The listing builds one solid part. Answer for the finished solid, in the listing's coordinates (mm). A direction names the side the tool comes from. Give positions to 0.01 mm unless a question says otherwise; leave off trailing zeros. Order: outer loops, then holes, each group sorted by start corner. A loop starts at its lowest first (then second) coordinate and runs counter-clockwise, first axis right, second up. Notation, with made-up numbers: (-16, 61) - (40, 61) arc R20 ccw to (40, 98) - close; hole circle Ø7 at (57.25, 89.5). An arc over 180 degrees is marked (long way). Write each question's results on one line, items separated by ' | '. Start each with the question number.
1. Find the intervals of material crossed by L1, parallel to X at y = 0.7, z = 0; L2, parallel to X at y = 2, z = 0; L3, parallel to Z at x = -8, y = 7.75, in increasing order.
2. Section B-B (y = 6.5) is taken. Give the vertices of the cut face in (x, z).
3. Section D-D (z = 5) is taken. Give the vertices of the cut face in (x, y) (3 decimals), and give its area (3 significant figures).
4. Section A-A (z = 0) is taken. State how many separate pieces and enclosed holes the cut face has, and give its area (3 significant figures).
5. Flat-ended cylindrical pins translate along their axes: pin 1 (1.3 mm diameter, centred on y = 7.5, z = -9.5, fed in from +X); pin 2 (4 mm diameter, centred on y = 5.5, z = 2, fed in from -X); pin 3 (1.3 mm diameter, centred on x = -3, z = -9.5, fed in from +Y) (3 decimals). Find the tip coordinate at first contact, or state that the pin passes through.
6. Section C-C (x = -4) is taken. Give the vertices of the cut face in (y, z) (1 decimal), and give its area (3 significant figures).
7. Which of the six approach directions +Z, -Z, +X, -X, +Y, -Y give full straight-line access (tool end or side, diameter ignored) to faces 1 (the face through (15.589, 8, 0)), 2 (the face through (0, 5, 10.033)), 3 (the face through (8.895, 7.254, -4.934)), 4 (the face through (11, 1.026, 0)), 5 (the face through (6.35, 8, 9))?
8. Determine the mould class of faces 6 (the face through (19, 0, 0)), 7 (the face through (-27.97, 1.288, -9.753)), 8 (the face through (16.353, 3.264, -0.14)), 9 (the face through (25.272, 1.288, 1.172)) for opening direction X: released by +X, released by -X, zero draft, split by the parting line, or undercut.
from build123d import *

# Parameters (mm, degrees)
SKETCH1_W               = 32.0675
SKETCH1_H               = 20.955
BOSS_EXTRUDE2_DEPTH     = 2.54
SKETCH3_W               = 31.1785
SKETCH3_H               = 20.066
SKETCH3_W_2             = 28.0035
SKETCH3_H_2             = 16.891
EXTRUDE_THIN1_DEPTH     = 8.255
CUT_EXTRUDE1_DEPTH      = 29.508335431
CUT_EXTRUDE1_DEPTH_BACK = 29.508335431
SKETCH4_W               = 12.7
SKETCH4_H               = 5.08
SKETCH5_R               = 1.5
BOSS_EXTRUDE3_DEPTH     = 8.255
FILLET1_R               = 1.27
CUT_EXTRUDE2_DEPTH      = 29.508335431
CUT_EXTRUDE2_DEPTH_BACK = 29.508335431
SKETCH6_W               = 3.048
SKETCH6_H               = 1.02616
SKETCH7_W               = 20.955
SKETCH7_H               = 2.54
BOSS_EXTRUDE4_DEPTH     = 12.7
FILLET2_R               = 2.54
FILLET3_R               = 2.54
SKETCH8_R               = 2.54
CUT_EXTRUDE3_DEPTH      = 32.67887972
FILLET4_R               = 2.54


with BuildPart() as part:
    # Sketch1 → Boss-Extrude2 (new body)
    with BuildSketch(Plane(origin=(0, 0, 0), x_dir=(1, 0, 0), z_dir=(0, 1, 0))):
        Rectangle(SKETCH1_W, SKETCH1_H)
    extrude(amount=BOSS_EXTRUDE2_DEPTH)

    # Sketch3 → Extrude-Thin1 (add)
    with BuildSketch(Plane(origin=(0, 2.54, 0), x_dir=(1, 0, 0), z_dir=(0, 1, 0))):
        Rectangle(SKETCH3_W, SKETCH3_H)
        Rectangle(SKETCH3_W_2, SKETCH3_H_2, mode=Mode.SUBTRACT)
    extrude(amount=EXTRUDE_THIN1_DEPTH)

    # Sketch4 → Cut-Extrude1 (cut, two sides: drawn at the far end of the back side and taken through both)
    with BuildSketch(Plane(origin=(0, 0, -10.4775), x_dir=(-1, 0, 0), z_dir=(0, 0, -1)).offset(-CUT_EXTRUDE1_DEPTH_BACK)):
        with Locations((0, 8.255)):
            Rectangle(SKETCH4_W, SKETCH4_H)
    extrude(amount=CUT_EXTRUDE1_DEPTH + CUT_EXTRUDE1_DEPTH_BACK, mode=Mode.SUBTRACT)

    # Sketch5 → Boss-Extrude3 (add)
    with BuildSketch(Plane(origin=(0, 2.54, 0), x_dir=(1, 0, 0), z_dir=(0, 1, 0))):
        with Locations(Location((-10.16, 4.1275, 0), (0, 0, 270))):
            Circle(SKETCH5_R)
        with Locations(Location((10.16, 4.1275, 0), (0, 0, 90))):
            Circle(SKETCH5_R)
    extrude(amount=BOSS_EXTRUDE3_DEPTH)

    # Fillet1
    fillet1_edges = [part.edges().sort_by_distance(p)[0] for p in [
        (-10.16, 2.54, -5.6275),
        (10.16, 2.54, -2.6275),
    ]]
    fillet(fillet1_edges, radius=FILLET1_R)

    # Sketch6 → Cut-Extrude2 (cut, two sides: drawn at the far end of the back side and taken through both)
    with BuildSketch(Plane.XY.offset(10.4775).offset(-CUT_EXTRUDE2_DEPTH_BACK)):
        with Locations((-10.969625, 0.51308)):
            Rectangle(SKETCH6_W, SKETCH6_H)
        with Locations((10.969625, 0.51308)):
            Rectangle(SKETCH6_W, SKETCH6_H)
    extrude(amount=CUT_EXTRUDE2_DEPTH + CUT_EXTRUDE2_DEPTH_BACK, mode=Mode.SUBTRACT)

    # Sketch7 → Boss-Extrude4 (add)
    with BuildSketch(Plane.ZY.offset(16.03375)):
        with Locations((0, 1.27)):
            Rectangle(SKETCH7_W, SKETCH7_H)
    boss_extrude4 = extrude(amount=BOSS_EXTRUDE4_DEPTH)

    # Fillet2
    fillet2_edges = [part.edges().sort_by_distance(p)[0] for p in [
        (-28.73375, 1.27, -10.4775),
        (-28.73375, 1.27, 10.4775),
    ]]
    fillet(fillet2_edges, radius=FILLET2_R)

    # Fillet3
    fillet3_edges = [part.edges().sort_by_distance(p)[0] for p in [
        (-15.58925, 2.54, 0),
    ]]
    fillet(fillet3_edges, radius=FILLET3_R)

    # Sketch8 → Cut-Extrude3 (cut, symmetric)
    with BuildSketch(Plane(origin=(0, 2.54, 0), x_dir=(1, 0, 0), z_dir=(0, 1, 0))):
        with Locations(Location((-23.01875, 0, 0), (0, 0, 270))):
            Circle(SKETCH8_R)
    cut_extrude3 = extrude(amount=CUT_EXTRUDE3_DEPTH, both=True, mode=Mode.SUBTRACT)

    # Mirror2: Boss-Extrude4 across plane
    add(boss_extrude4.mirror(Plane(origin=(0, 0, 0), x_dir=(0, 0, 1), z_dir=(1, 0, 0))))

    # Mirror6: Cut-Extrude3 across plane
    add(cut_extrude3.mirror(Plane(origin=(0, 0, 0), x_dir=(0, 0, 1), z_dir=(1, 0, 0))), mode=Mode.SUBTRACT)

    # Fillet4
    fillet4_edges = [part.edges().sort_by_distance(p)[0] for p in [
        (28.73375, 1.27, -10.4775),
        (28.73375, 1.27, 10.4775),
        (15.58925, 2.54, 0),
    ]]
    fillet(fillet4_edges, radius=FILLET4_R)


solid = part.part
Reported:
1) L1: -28.73 to -25.56, -20.48 to -12.49, -9.45 to 9.45, 12.49 to 20.48, 25.56 to 28.73 | L2: -28.73 to -25.56, -20.48 to 20.48, 25.56 to 28.73 | L3: -10.03 to -8.45, 8.45 to 10.03
2) outline: (-15.59, -10.03) - (-6.35, -10.03) - (-6.35, -8.45) - (-14, -8.45) - (-14, 8.45) - (-6.35, 8.45) - (-6.35, 10.03) - (-15.59, 10.03) - close; circle Ø3 at (-10.16, -4.13); (6.35, -10.03) - (15.59, -10.03) - (15.59, 10.03) - (6.35, 10.03) - (6.35, 8.45) - (14, 8.45) - (14, -8.45) - (6.35, -8.45) - close; circle Ø3 at (10.16, -4.13)
3) outline: (-28.734, 0) - (-12.494, 0) - (-12.494, 1.026) - (-9.446, 1.026) - (-9.446, 0) - (9.446, 0) - (9.446, 1.026) - (12.494, 1.026) - (12.494, 0) - (28.734, 0) - (28.734, 2.54) - (18.129, 2.54) arc R2.54 cw to (15.589, 5.08) - (15.589, 10.795) - (14.002, 10.795) - (14.002, 2.54) - (-14.002, 2.54) - (-14.002, 10.795) - (-15.589, 10.795) - (-15.589, 5.08) arc R2.54 cw to (-18.129, 2.54) - (-28.734, 2.54) - close | area: 169 mm²
4) separate pieces: 3 | enclosed holes: 0 | area: 143 mm²
5) pin 1: x = 15.59 | pin 2: x = -16.14 | pin 3: y = 5.715
6) outline: (0, -10.5) - (2.5, -10.5) - (2.5, -10) - (5.7, -10) - (5.7, -8.4) - (2.5, -8.4) - (2.5, 8.4) - (5.7, 8.4) - (5.7, 10) - (2.5, 10) - (2.5, 10.5) - (0, 10.5) - close | area: 63.3 mm²
7) face 1: +Z, -Z, +X, +Y | face 2: +Z, +X, -X, +Y | face 3: +Y | face 4: +Z, -Z, -Y | face 5: +Z, -Z, +Y
8) face 6: zero draft | face 7: released by -X | face 8: released by +X | face 9: undercut
